Work out the finished part from the listing and answer in its coordinate system (mm). A direction names the side the tool comes from. Give positions to 0.01 mm unless a question says otherwise; leave off trailing zeros. Loops run counter-clockwise (first coordinate to the right, second up) from the corner with the lowest first, then second, coordinate; pieces in that order, holes last. Notation, with made-up numbers: (68, 28) -> (109, 28) arc R21 ccw to (109, 53) -> close; hole circle Ø11 at (62, 31.5). An arc over 180 degrees is marked (long way). Answer as CSV lines item,"result". Start each with the question number.
1. Determine the mould class of faces 3 (the face through (13, 84, 0)), 4 (the face through (25.4, 81, 13)), 5 (the face through (14.04, 65.6, 24.15)) for opening direction X: +X half, -X half, draft (parallel to the pull), parting line (faces both ways), or undercut.
2. Find section B-B, the plane y = 152.91. Give the vertices of the cut face in (x, z), and give its area (3 significant figures).
3. Find section D-D, the plane y = 25. Give the vertices of the cut face in (x, z).
4. Find section A-A, the plane z = 9.5. Give the vertices of the cut face in (x, y).
5. A flat-ended cylindrical pin translates along its axis: pin 1 Ø4 at (x, y) = (12.7, 44.45) entering from -Z. Find the tip coordinate at first contact, or state that the pin passes through.
6. Find section C-C, the plane x = 17. Give the vertices of the cut face in (y, z).
7. A tool of negligible diameter and unlimited length cuts with its end or side. For faces 1 (the face through (15.363, 10.759, 1.288)), 2 (the face through (22.86, 84, 13)), from which of +Z, -Z, +X, -X, +Y, -Y can it reach the whole face along a straight path? Write none if from no direction.
8. Find the intervals of material crossed by line 1 along X through (y, z) = (148.5, 19.5); line 2 along Y through (x, z) = (8.5, 24.25), in increasing order.
from build123d import *

# Parameters (mm, degrees)
SKETCH1_W           = 25.4
SKETCH1_H           = 165.1
BOSS_EXTRUDE1_DEPTH = 25.4
SKETCH2_W           = 20.32
SKETCH2_H           = 20.32
CUT_EXTRUDE1_DEPTH  = 166.1
SKETCH4_R           = 4.7625
CUT_EXTRUDE2_DEPTH  = 26.4
SKETCH8_R           = 2.4892
SKETCH8_R_2         = 2.413
CUT_EXTRUDE4_DEPTH  = 26.4


with BuildPart() as part:
    # Sketch1 → Boss-Extrude1 (new body)
    with BuildSketch(Plane.XY):
        with Locations((12.7, 82.55)):
            Rectangle(SKETCH1_W, SKETCH1_H)
    extrude(amount=BOSS_EXTRUDE1_DEPTH)

    # Sketch2 → Cut-Extrude1 (cut, through all)
    with BuildSketch(Plane(origin=(0, 165.1, 0), x_dir=(1, 0, 0), z_dir=(0, 1, 0))):
        with Locations((12.7, -12.7)):
            Rectangle(SKETCH2_W, SKETCH2_H)
    extrude(amount=-CUT_EXTRUDE1_DEPTH, mode=Mode.SUBTRACT)

    # Sketch4 → Cut-Extrude2 (cut, through all)
    with BuildSketch(Plane.XY.offset(25.4)):
        with Locations((10.82039492, 152.91000025)):
            Circle(SKETCH4_R)
    cut_extrude2 = extrude(amount=-CUT_EXTRUDE2_DEPTH, mode=Mode.SUBTRACT)

    # Mirror1: Cut-Extrude2 across plane
    add(cut_extrude2.mirror(Plane.ZX.offset(82.55)), mode=Mode.SUBTRACT)

    # Sketch8 → Cut-Extrude4 (cut, through all)
    with BuildSketch(Plane.XY.offset(25.4)):
        with Locations((12.7, 63.5)):
            Circle(SKETCH8_R)
        with Locations((12.7, 44.45)):
            Circle(SKETCH8_R_2)
        with Locations((16.419743879, 35.469743879)):
            Circle(SKETCH8_R)
        with Locations((12.7, 101.6)):
            Circle(SKETCH8_R)
        with Locations((12.7, 120.65)):
            Circle(SKETCH8_R_2)
        with Locations((16.419743879, 129.630256121)):
            Circle(SKETCH8_R)
    extrude(amount=-CUT_EXTRUDE4_DEPTH, mode=Mode.SUBTRACT)


solid = part.part
Resolved:
1,face 3,"draft"
1,face 4,"+X half"
1,face 5,"undercut"
2,outline,"(0, 0) -> (6.06, 0) -> (6.06, 2.54) -> (2.54, 2.54) -> (2.54, 22.86) -> (6.06, 22.86) -> (6.06, 25.4) -> (0, 25.4) -> close; (15.58, 0) -> (25.4, 0) -> (25.4, 25.4) -> (15.58, 25.4) -> (15.58, 22.86) -> (22.86, 22.86) -> (22.86, 2.54) -> (15.58, 2.54) -> close"
2,area,"184 mm^2"
3,outline,"(0, 0) -> (25.4, 0) -> (25.4, 25.4) -> (0, 25.4) -> close; hole (2.54, 2.54) -> (22.86, 2.54) -> (22.86, 22.86) -> (2.54, 22.86) -> close"
4,outline,"(0, 0) -> (2.54, 0) -> (2.54, 165.1) -> (0, 165.1) -> close; (22.86, 0) -> (25.4, 0) -> (25.4, 165.1) -> (22.86, 165.1) -> close"
5,pin 1,"passes through"
6,outline,"(0, 0) -> (33.05, 0) -> (33.05, 2.54) -> (0, 2.54) -> close; (0, 22.86) -> (33.05, 22.86) -> (33.05, 25.4) -> (0, 25.4) -> close; (37.89, 0) -> (127.21, 0) -> (127.21, 2.54) -> (37.89, 2.54) -> close; (37.89, 22.86) -> (127.21, 22.86) -> (127.21, 25.4) -> (37.89, 25.4) -> close; (132.05, 0) -> (165.1, 0) -> (165.1, 2.54) -> (132.05, 2.54) -> close; (132.05, 22.86) -> (165.1, 22.86) -> (165.1, 25.4) -> (132.05, 25.4) -> close"
7,face 1,"+Z, -Z"
7,face 2,"+Y, -Y"
8,line 1,"x = 0 to 2.54, 22.86 to 25.4"
8,line 2,"y = 0 to 8.03, 16.35 to 148.75, 157.07 to 165.1"
